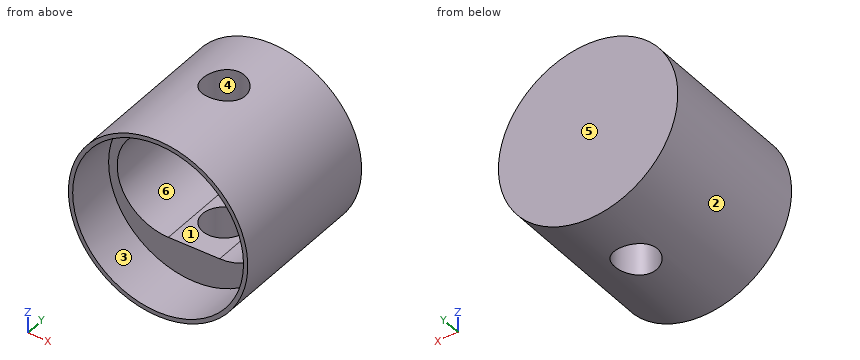
from build123d import *

# Parameters (mm, degrees)
SKETCH1_R               = 10.5
BOSS_EXTRUDE1_DEPTH     = 19
SKETCH2_R               = 10
CUT_EXTRUDE1_DEPTH      = 6
CUT_EXTRUDE2_DEPTH      = 11
CUT_EXTRUDE3_DEPTH      = 25.114311104
CUT_EXTRUDE3_DEPTH_BACK = 25.114311104
SKETCH4_R               = 2.5


with BuildPart() as part:
    # Sketch1 → Boss-Extrude1 (new body)
    with BuildSketch(Plane(origin=(0, 0, 0), x_dir=(1, 0, 0), z_dir=(0, 1, 0))):
        with Locations(Location((0, 0, 0), (0, 0, 270))):
            Circle(SKETCH1_R)
    extrude(amount=BOSS_EXTRUDE1_DEPTH)

    # Sketch2 → Cut-Extrude1 (cut)
    with BuildSketch(Plane.XZ):
        with Locations(Location((0, 0, 0), (0, 0, 270))):
            Circle(SKETCH2_R)
    extrude(amount=-CUT_EXTRUDE1_DEPTH, mode=Mode.SUBTRACT)

    # Sketch3 → Cut-Extrude2 (cut)
    with BuildSketch(Plane.XZ.offset(-6)):
        with BuildLine():
            Line((3, -6), (-3, -6))
            ThreePointArc((-3, -6), (-9, 0), (-3, 6))
            Line((-3, 6), (3, 6))
            ThreePointArc((3, 6), (9, 0), (3, -6))
        make_face()
    extrude(amount=-CUT_EXTRUDE2_DEPTH, mode=Mode.SUBTRACT)

    # Sketch4 → Cut-Extrude3 (cut, two sides: drawn at the far end of the back side and taken through both)
    with BuildSketch(Plane.XY.offset(-CUT_EXTRUDE3_DEPTH_BACK)):
        with Locations((0, 11)):
            Circle(SKETCH4_R)
    extrude(amount=CUT_EXTRUDE3_DEPTH + CUT_EXTRUDE3_DEPTH_BACK, mode=Mode.SUBTRACT)


solid = part.part
Work out the finished part from the listing and answer in its coordinate system (mm). Face numbers are marked on the shaded views. A direction names the side the tool comes from. Coordinates: 2 decimals unless noted, no trailing zeros. Write each loop counter-clockwise with the first axis right and the second up, starting at its lowest first coordinate (ties: lowest second). Pieces come first, ordered by that corner, then holes. Notation, with made-up numbers: M 6.25,87 L 65.25,87 A10 cw 65.25,96 Z; hole C 1,-29 d10. An arc over 180 degrees is marked long. Answer as CSV lines item,"result". Start each with the question number.
Item 1: Section C-C on z = 7 is taken. Write down the section's boundary in (x, y).
Item 2: Consider L1, parallel to X at y = 1.95, z = 0; L2, parallel to Y at x = -6.75, z = -2.25; L3, parallel to Z at x = 5.25, y = 6.75. Determine where each line is inside the solid, lowest interval first.
Item 3: Section B-B on y = 11 is taken. Write down the section's boundary in (x, z), and give its area (3 significant figures).
Item 4: Section D-D on z = 0 is taken. Write down the section's boundary in (x, y).
Item 5: Section A-A on x = 0 is taken. Write down the section's boundary in (y, z).
Item 6: Flat-ended cylindrical pins translate along their axes: P1, Ø10, axis at y = 8.5, z = -7.5, coming from the -X side; P2, Ø6, axis at x = -3.5, y = 3.5, coming from the -Z side; P3, Ø4, axis at x = 3, z = 1.5, coming from the -Y side. Find the tip coordinate at first contact, or state that the pin passes through.
Item 7: Determine the mould class of the marked faces 1, 2, 3 and 4 for opening direction Z: released by +Z, released by -Z, zero draft, split by the parting line, or undercut.
Item 8: A tool of negligible diameter and unlimited length cuts with its end or side. For the marked faces 5 and 6, from which of +Z, -Z, +X, -X, +Y, -Y can it reach the whole face along a straight path? Write none if from no direction.
Checks:
1,outline,"M -7.83,0 L -7.14,0 L -7.14,6 L 7.14,6 L 7.14,0 L 7.83,0 L 7.83,19 L -7.83,19 Z; hole C 0,11 d5"
2,L1,"x = -10.5 to -10, 10 to 10.5"
2,L2,"y = 17 to 19"
2,L3,"z = -9.09 to -5.56, 5.56 to 9.09"
3,outline,"M -3,-6 A6 cw -3,6 L -2.5,6 L -2.5,10.2 A10.5 ccw -2.5,-10.2 L -2.5,-6 Z; M 2.5,-10.2 A10.5 ccw 2.5,10.2 L 2.5,6 L 3,6 A6 cw 3,-6 L 2.5,-6 Z"
3,area,"117 mm²"
4,outline,"M -10.5,0 L -10,0 L -10,6 L -9,6 L -9,17 L 9,17 L 9,6 L 10,6 L 10,0 L 10.5,0 L 10.5,19 L -10.5,19 Z"
5,outline,"M 0,-10.5 L 8.5,-10.5 L 8.5,-6 L 6,-6 L 6,-10 L 0,-10 Z; M 0,10 L 6,10 L 6,6 L 8.5,6 L 8.5,10.5 L 0,10.5 Z; M 13.5,-10.5 L 19,-10.5 L 19,10.5 L 13.5,10.5 L 13.5,6 L 17,6 L 17,-6 L 13.5,-6 Z"
6,P1,"stops at x = -10.2"
6,P2,"stops at z = -10.49"
6,P3,"stops at y = 17"
7,face 1,"undercut"
7,face 2,"split by the parting line"
7,face 3,"undercut"
7,face 4,"zero draft"
8,face 5,"+Z, -Z, +X, -X, +Y"
8,face 6,"-Y"
